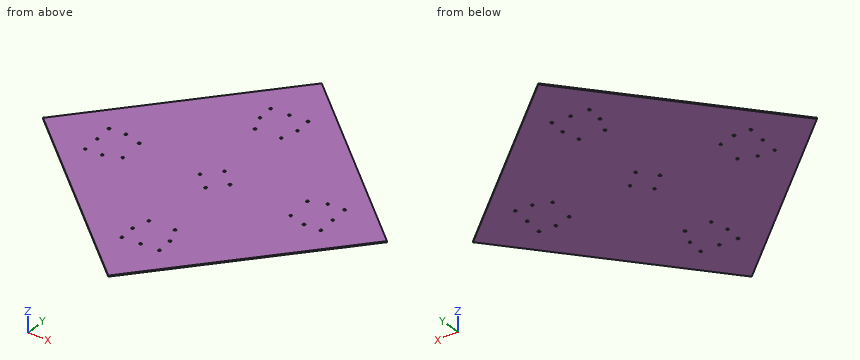
from build123d import *

# Parameters (mm, degrees)
BOSS_EXTRUDE1_DEPTH     = 3
CUT_EXTRUDE1_DEPTH      = 2677.124530624
CUT_EXTRUDE1_DEPTH_BACK = 2677.124530624
SKETCH2_R               = 3
SKETCH2_R_2             = 3.3
SKETCH2_R_3             = 3.25


with BuildPart() as part:
    # Sketch1 → Boss-Extrude1 (new body)
    with BuildSketch(Plane.XY):
        Polygon((964.746903845, -1307.864551018), (551.817114678, -1803.358233337), (1064.979563964, -2231.012650645), (1477.909353131, -1735.518968326), align=None)
    extrude(amount=BOSS_EXTRUDE1_DEPTH)

    # Sketch2 → Cut-Extrude1 (cut, two sides: drawn at the far end of the back side and taken through both)
    with BuildSketch(Plane.XY.offset(3).offset(-CUT_EXTRUDE1_DEPTH_BACK)):
        with Locations((794.552341263, -1824.606259686)):
            Circle(SKETCH2_R)
        with Locations((701.753786497, -1797.896182314)):
            Circle(SKETCH2_R)
        with Locations((706.279483297, -1847.690941762)):
            Circle(SKETCH2_R)
        with Locations((751.0947668, -1843.617814641)):
            Circle(SKETCH2_R)
        with Locations((697.228089696, -1748.101422866)):
            Circle(SKETCH2_R_2)
        with Locations((742.043373199, -1744.028295746)):
            Circle(SKETCH2_R_2)
        with Locations((788.216365742, -1754.893596459)):
            Circle(SKETCH2_R_2)
        with Locations((1054.699041463, -1765.818043391)):
            Circle(SKETCH2_R_3)
        with Locations((1011.242676464, -1729.602793273)):
            Circle(SKETCH2_R_3)
        with Locations((975.027426346, -1773.059158272)):
            Circle(SKETCH2_R_3)
        with Locations((1018.483791345, -1809.27440839)):
            Circle(SKETCH2_R_3)
        with Locations((959.695575049, -1549.12770819)):
            Circle(SKETCH2_R_2)
        with Locations((940.684020094, -1505.670133727)):
            Circle(SKETCH2_R_2)
        with Locations((936.610892974, -1460.854850224)):
            Circle(SKETCH2_R_2)
        with Locations((986.405652422, -1456.329153423)):
            Circle(SKETCH2_R_2)
        with Locations((1036.200411869, -1451.803456623)):
            Circle(SKETCH2_R_2)
        with Locations((1040.27353899, -1496.618740126)):
            Circle(SKETCH2_R_2)
        with Locations((1029.408238276, -1542.791732669)):
            Circle(SKETCH2_R_2)
        with Locations((993.52605594, -2087.07374504)):
            Circle(SKETCH2_R_2)
        with Locations((1043.320815388, -2082.548048239)):
            Circle(SKETCH2_R_2)
        with Locations((989.452928819, -2042.258461537)):
            Circle(SKETCH2_R_2)
        with Locations((1000.318229533, -1996.085468994)):
            Circle(SKETCH2_R_2)
        with Locations((1070.03089276, -1989.749493473)):
            Circle(SKETCH2_R_2)
        with Locations((1089.042447715, -2033.207067936)):
            Circle(SKETCH2_R_2)
        with Locations((1093.115574835, -2078.022351439)):
            Circle(SKETCH2_R_2)
        with Locations((1241.510102067, -1783.983605203)):
            Circle(SKETCH2_R_2)
        with Locations((1287.68309461, -1794.848905917)):
            Circle(SKETCH2_R_2)
        with Locations((1332.498378113, -1790.775778796)):
            Circle(SKETCH2_R_2)
        with Locations((1327.972681313, -1740.981019348)):
            Circle(SKETCH2_R_2)
        with Locations((1323.446984512, -1691.186259901)):
            Circle(SKETCH2_R_2)
        with Locations((1278.631701009, -1695.259387021)):
            Circle(SKETCH2_R_2)
        with Locations((1235.174126546, -1714.270941976)):
            Circle(SKETCH2_R_2)
    extrude(amount=CUT_EXTRUDE1_DEPTH + CUT_EXTRUDE1_DEPTH_BACK, mode=Mode.SUBTRACT)


solid = part.part
The listing builds one solid part. Answer for the finished solid, in the listing's coordinates (mm). Coordinates: 2 decimals unless noted, no trailing zeros. Write each loop counter-clockwise with the first axis right and the second up, starting at its lowest first coordinate (ties: lowest second). Pieces come first, ordered by that corner, then holes. Notation, with made-up numbers: (-5.75, 44) - (8.25, 44) arc R8 cw to (8.25, 54) - close; hole circle Ø1 at (28, 80.25). An arc over 180 degrees is marked (long way). Return JSON: item names as keys, results as strings.
1. The part is cut by section A-A on z = 0.45. Count the separate pieces of the cut face and the enclosed holes in it, then the cut area to 3 significant figures.
Final values:
{"separate pieces": "1", "enclosed holes": "32", "area": "430,000 mm^2"}
2. The part is cut by section B-B on y = -1662.5. Determine the outline of the cut face in (x, z).
Final values:
{"outline": "(669.2, 0) - (1390.29, 0) - (1390.29, 3) - (669.2, 3) - close"}
3. The part is cut by section C-C on x = 1415. Determine the outline of the cut face in (y, z), then the cut area to 3 significant figures.
Final values:
{"outline": "(-1811.01, 0) - (-1683.09, 0) - (-1683.09, 3) - (-1811.01, 3) - close", "area": "384 mm^2"}
4. Each of these flat-tipped pins is pushed along its axis until it touches: pin 1 Ø5.5 at (x, y) = (936.61, -1460.85) entering from -Z; pin 2 Ø1 at (y, z) = (-1932, 1) entering from +X. Where does it stop, or does it pass through?
Final values:
{"pin 1": "through", "pin 2": "x = 1314.58"}
5. Consider line 1 along Y through (x, z) = (990.5, 2.35); line 2 along Y through (x, z) = (988.5, 0.45); line 3 along X through (y, z) = (-1800.5, 1.25). Determine where each line is inside the solid, lowest interval first.
Final values:
{"line 1": "-2168.94 to -2088.39, -2085.76 to -2045.39, -2039.13 to -1329.33", "line 2": "-2167.28 to -2045.42, -2039.1 to -1458.88, -1453.78 to -1327.66", "line 3": "554.2 to 700.26, 703.24 to 1423.76"}
